Design review of the part built by this model. Coordinates are the model's own, in mm. Round coordinates to 2 decimals unless told otherwise and drop trailing zeros. Loops run counter-clockwise (first coordinate to the right, second up) from the corner with the lowest first, then second, coordinate; pieces in that order, holes last. Notation, with made-up numbers: (-1.75, 62.25) - (15.25, 62.25) arc R25 ccw to (15.25, 77.25) - close; hole circle Ø7 at (68, -11). An arc over 180 degrees is marked (long way). Return JSON: item names as keys, results as strings. Group by question number.
(1) Wall thickness on L1, parallel to Z at x = -0.45, y = -1.7; L2, parallel to Z at x = 1.2, y = -1.45; L3, parallel to X at y = 0.05, z = 9: over which ranges is each line inside the solid? List them lowest first. Write a range as [from, to].
(2) We need section C-C, the plane z = 4.25. Write out the cut boundary in (x, y).
(3) We need section A-A, the plane x = 0. Write out the cut boundary in (y, z), and give its area (3 significant figures).
(4) The part is to be moulded in two halves that separate along Z. For faces 1 (the cylindrical face through (-1.5, 0.07, 8.63)), 2 (the flat face through (0, 0, 18.5)), 3 (the cylindrical face through (0.434, -1.952, -0.246)), say which applies: pulls with the +Z half, pulls with the -Z half, needs draft (parallel to the pull), parting line crosses it, or undercut.
from build123d import *

# Parameters (mm, degrees)
SKETCH1_R           = 1.5
BOSS_EXTRUDE1_DEPTH = 17.5
SKETCH2_R           = 2
BOSS_EXTRUDE2_DEPTH = 1
SKETCH3_R           = 2
BOSS_EXTRUDE3_DEPTH = 1
FILLET1_R           = 0.5


with BuildPart() as part:
    # Sketch1 → Boss-Extrude1 (new body)
    with BuildSketch(Plane.XY):
        Circle(SKETCH1_R)
    extrude(amount=BOSS_EXTRUDE1_DEPTH)

    # Sketch2 → Boss-Extrude2 (add)
    with BuildSketch(Plane(origin=(0, 0, 0), x_dir=(-1, 0, 0), z_dir=(0, 0, -1))):
        Circle(SKETCH2_R)
    extrude(amount=BOSS_EXTRUDE2_DEPTH)

    # Sketch3 → Boss-Extrude3 (add)
    with BuildSketch(Plane.XY.offset(17.5)):
        Circle(SKETCH3_R)
    extrude(amount=BOSS_EXTRUDE3_DEPTH)

    # Fillet1
    fillet1_edges = [part.edges().sort_by_distance(p)[0] for p in [
        (-2, 0, 18.5),
        (2, 0, -1),
    ]]
    fillet(fillet1_edges, radius=FILLET1_R)


solid = part.part
Solutions:
{
 "1": {"L1": "[-0.93, 0], [17.5, 18.43]", "L2": "[-0.82, 0], [17.5, 18.32]", "L3": "[-1.5, 1.5]"},
 "2": {"outline": "circle Ø3 at (0, 0)"},
 "3": {"outline": "(-2, -0.5) arc R0.5 ccw to (-1.5, -1) - (1.5, -1) arc R0.5 ccw to (2, -0.5) - (2, 0) - (1.5, 0) - (1.5, 17.5) - (2, 17.5) - (2, 18) arc R0.5 ccw to (1.5, 18.5) - (-1.5, 18.5) arc R0.5 ccw to (-2, 18) - (-2, 17.5) - (-1.5, 17.5) - (-1.5, 0) - (-2, 0) - close", "area": "60.3 mm^2"},
 "4": {"face 1": "undercut", "face 2": "pulls with the +Z half", "face 3": "needs draft"}
}
